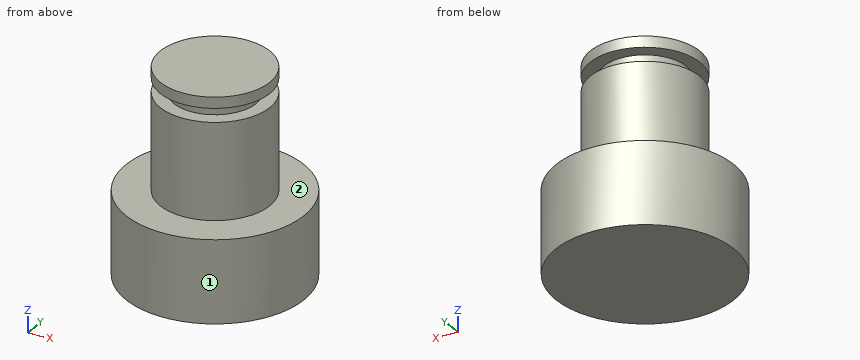
```python
from build123d import *

# Parameters (mm, degrees)
SKETCH1_R           = 6.5
BOSS_EXTRUDE1_DEPTH = 6
SKETCH2_R           = 4
BOSS_EXTRUDE2_DEPTH = 8.8
SKETCH3_R           = 4
SKETCH3_R_2         = 3
CUT_EXTRUDE1_DEPTH  = 0.5


with BuildPart() as part:
    # Sketch1 → Boss-Extrude1 (new body)
    with BuildSketch(Plane.XY):
        Circle(SKETCH1_R)
    extrude(amount=-BOSS_EXTRUDE1_DEPTH)

    # Sketch2 → Boss-Extrude2 (add)
    with BuildSketch(Plane.XY):
        Circle(SKETCH2_R)
    extrude(amount=BOSS_EXTRUDE2_DEPTH)

    # Sketch3 → Cut-Extrude1 (cut, symmetric)
    with BuildSketch(Plane.XY.offset(7.5)):
        Circle(SKETCH3_R)
        Circle(SKETCH3_R_2, mode=Mode.SUBTRACT)
    extrude(amount=CUT_EXTRUDE1_DEPTH, both=True, mode=Mode.SUBTRACT)


solid = part.part
```
The listing builds one solid part. Answer for the finished solid, in the listing's coordinates (mm). Face numbers are marked on the shaded views. A direction names the side the tool comes from. Coordinates: 2 decimals unless noted, no trailing zeros. Write each loop counter-clockwise with the first axis right and the second up, starting at its lowest first coordinate (ties: lowest second). Pieces come first, ordered by that corner, then holes.
Q1. Given P1, Ø1, axis at x = 3, z = 4, coming from the -Y side; P2, Ø4, axis at x = 3.5, z = -2.5, coming from the -Y side; P3, Ø5, axis at y = -4.5, z = -1.5, coming from the -X side, each flat-ended and moving along its own axis, determine where each tip first touches the part or whether it passes through.
Returned:
P1: stops at y = -3.12
P2: stops at y = -6.32
P3: stops at x = -6.18
Q2. Which of the six approach directions +Z, -Z, +X, -X, +Y, -Y give full straight-line access (tool end or side, diameter ignored) to the marked faces 1 and 2?
Returned:
face 1: +Z, -Z
face 2: +Z
Q3. Section D-D, the plane z = -0.5 is taken. Write down the section's boundary in (x, y).
Returned:
outline: circle Ø13 at (0, 0)
Q4. Section C-C, the plane y = -3.75 is taken. Write down the section's boundary in (x, z), then the cut area to 3 significant figures.
Returned:
outline: (-5.31, -6) - (5.31, -6) - (5.31, 0) - (1.39, 0) - (1.39, 7) - (-1.39, 7) - (-1.39, 0) - (-5.31, 0) - close; (-1.39, 8) - (1.39, 8) - (1.39, 8.8) - (-1.39, 8.8) - close
area: 85.4 mm2
Q5. Find the intervals of material crossed by line 1 along Z through (x, y) = (-3, 2.25); line 2 along X through (y, z) = (0.25, -2); line 3 along Y through (x, z) = (-1.5, -1.75), in increasing order.
Returned:
line 1: z = -6 to 7, 8 to 8.8
line 2: x = -6.5 to 6.5
line 3: y = -6.32 to 6.32
Q6. Section A-A, the plane y = 0 is taken. Write down the section's boundary in (x, z), then the cut area to 3 significant figures.
Returned:
outline: (-6.5, -6) - (6.5, -6) - (6.5, 0) - (4, 0) - (4, 7) - (3, 7) - (3, 8) - (4, 8) - (4, 8.8) - (-4, 8.8) - (-4, 8) - (-3, 8) - (-3, 7) - (-4, 7) - (-4, 0) - (-6.5, 0) - close
area: 146 mm2
